The listing builds one solid part. Answer for the finished solid, in the listing's coordinates (mm). A direction names the side the tool comes from. Round coordinates to 2 decimals unless told otherwise and drop trailing zeros. Write each loop counter-clockwise with the first axis right and the second up, starting at its lowest first coordinate (ties: lowest second). Pieces come first, ordered by that corner, then holes. Notation, with made-up numbers: M 18.5,-39 L 50.5,-39 A16 cw 50.5,-18 Z; hole C 26,-38 d3. An arc over 180 degrees is marked long. One line per item, written item: value. Start each with the question number.
(1) Section A-A (z = -42.1) is taken. Determine the outline of the cut face in (x, y).
(2) Given P1, Ø1, axis at x = 38, y = -25.5, coming from the -Z side; P2, Ø5, axis at y = -10.47, z = -9.9, coming from the +X side; P3, Ø5, axis at y = -10.47, z = -42.1, coming from the -X side, each flat-ended and moving along its own axis, determine where each tip first touches the part or whether it passes through.
(3) For a pull along X with two mould halves and no side action, classify faces 3 (the flat face through (21, -16, 2)), 4 (the cylindrical face through (35.57, -17.356, 0.986)), 5 (the flat face through (-12.504, -21, -26)), 6 (the flat face through (54.496, -16, 1)) as released by +X, released by -X, zero draft, split by the parting line, or undercut.
(4) Section B-B (z = -26) is taken. Determine the outline of the cut face in (x, y), plus the area to 3 significant figures.
(5) Section C-C (y = -33.5) is taken. Determine the outline of the cut face in (x, z), plus the area to 3 significant figures.
(6) Section D-D (x = 39) is taken. Determine the outline of the cut face in (y, z), plus the area to 3 significant figures.
(7) Consider probe 1 along Y at (x, z) = (-11.1, -42.1); probe 2 along Z at (x, y) = (26, -6.5); probe 3 along X at (y, z) = (-27.5, -40.5). Determine where each line is inside the solid, lowest interval first.
(8) For faces 1 (the cylindrical face through (-11.49, -9.896, -40.714)), 2 (the flat face through (-10.504, -21, -27)), determine the directions among +Z, -Z, +X, -X, +Y, -Y from which every point of the face is accessible in a straight line to the end or side of a thin tool.
Autodesk Inventor part; units mm, degrees
ref_plane "YZ Plane" through (0, 0, 0) normal (1, 0, 0) x (0, 1, 0)
ref_plane "XZ Plane" through (0, 0, 0) normal (0, 1, 0) x (-1, 0, 0)
ref_plane "XY Plane" through (0, 0, 0) normal (0, 0, 1) x (1, 0, 0)
sketch "スケッチ1" plane through (0, 0, 0) normal (0, 0, 1) x (1, 0, 0)
  line L0 (-10.5043, 6.5297) -> (54.4957, 6.5297)
  line L1 (54.4957, 6.5297) -> (54.4957, -38.4703)
  line L2 (54.4957, -38.4703) -> (-10.5043, -38.4703)
  line L3 (-10.5043, -38.4703) -> (-10.5043, 6.5297)
  point P0 (0, 0)
  dimension "d0" = 65
  dimension "d1" = 45
extrude "押し出し1" add sketch "スケッチ1" along normal blind 2
sketch "スケッチ2" plane through (-10.5043, -38.4703, 0) normal (-1, 0, 0) x (0, 0, 1)
  line L0 (-53, 45) -> (2, 45)
  line L1 (2, 45) -> (2, 0)
  line L2 (2, 0) -> (-53, 0)
  line L3 (-53, 0) -> (-53, 45)
  point P0 (0, 38.4703)
  point P1 (2, 45)
  dimension "d4" = 55
  dimension "d5" = 45
extrude "押し出し2" add sketch "スケッチ2" along normal blind 2
sketch "スケッチ3" plane through (-12.5043, -38.4703, 0) normal (-1, 0, 0) x (0, 0, 1)
  circle A0 centre (-26, 28) radius 6.3
  line L0 (2, 45) -> (-53, 45)
  line L1 (-53, 0) -> (2, 0)
  line L2 (-53, 45) -> (-53, 0)
  point P0 (0, 38.4703)
  dimension "d8" = 12.6
  dimension "d10" = 28
  dimension "d11" = 27
extrude "押し出し3" cut sketch "スケッチ3" against normal blind 2
sketch "スケッチ4" plane through (-12.5043, -38.4703, 0) normal (-1, 0, 0) x (0, 0, 1)
  circle A0 centre (-42.1, 28) radius 1.5
  circle A1 centre (-26, 28) radius 6.3
  line L0 (-53, 0) -> (2, 0)
  circle A2 centre (-9.9, 28) radius 1.5
  point P0 (0, 38.4703)
  dimension "d14" = 3
  dimension "d15" = 16.1
  dimension "d16" = 28
  dimension "d17" = 3
  dimension "d18" = 16.1
hole "穴1" at (-12.5043, -10.4703, -42.1) at (-12.5043, -10.4703, -9.9) direction (1, 0, 0) diameter 3 depth 2
sketch "スケッチ5" plane through (0, 0, 2) normal (0, 0, 1) x (1, 0, 0)
  circle A0 centre (44.9957, -15.9703) radius 1.5
  line L0 (54.4957, -38.4703) -> (54.4957, 6.5297)
  line L1 (54.4957, 6.5297) -> (-12.5043, 6.5297)
  circle A1 centre (34.9957, -15.9703) radius 1.5
  circle A2 centre (24.9957, -15.9703) radius 1.5
  point P0 (0, 0)
  dimension "d26" = 3
  dimension "d27" = 9.5
  dimension "d28" = 22.5
  dimension "d29" = 3
  dimension "d30" = 3
  dimension "d31" = 10
  dimension "d32" = 10
hole "穴2" at (24.9957, -15.9703, 2) at (34.9957, -15.9703, 2) at (44.9957, -15.9703, 2) direction (0, 0, -1) diameter 3 depth 2
equation "\"BendRadius\" = Thickness"
equation "\"BendReliefWidth\" = Thickness"
equation "\"BendReliefDepth\" = 0.5 * Thickness"
equation "\"CornerReliefSize\" = 4 * Thickness"
equation "\"MinimumRemnant\" = 2 * Thickness"
equation "\"TransitionRadius\" = BendRadius"
equation "\"JacobiRadiusSize\" = BendRadius"
equation "\"GapSize\" = Thickness"
properties part number "nhk16" material "アルミニウム 6061"
Recorded:
1. outline: M -12.5,-38.47 L -10.5,-38.47 L -10.5,-11.97 L -12.5,-11.97 Z; M -12.5,-8.97 L -10.5,-8.97 L -10.5,6.53 L -12.5,6.53 Z
2. P1: stops at z = 0
2. P2: stops at x = -10.5
2. P3: stops at x = -12.5
3. face 3: zero draft
3. face 4: undercut
3. face 5: released by -X
3. face 6: released by +X
4. outline: M -12.5,-38.47 L -10.5,-38.47 L -10.5,-16.77 L -12.5,-16.77 Z; M -12.5,-4.17 L -10.5,-4.17 L -10.5,6.53 L -12.5,6.53 Z
4. area: 64.8 mm2
5. outline: M -12.5,-53 L -10.5,-53 L -10.5,0 L 54.5,0 L 54.5,2 L -12.5,2 Z
5. area: 240 mm2
6. outline: M -38.47,0 L 6.53,0 L 6.53,2 L -38.47,2 Z
6. area: 90.0 mm2
7. probe 1: y = -38.47 to -11.97, -8.97 to 6.53
7. probe 2: z = 0 to 2
7. probe 3: x = -12.5 to -10.5
8. face 1: +X, -X
8. face 2: -Z, +X, +Y, -Y
